The model under review builds one solid part; all positions refer to its coordinate system, in mm. A direction names the side the tool comes from. Coordinates: 2 decimals unless noted, no trailing zeros. Loops run counter-clockwise (first coordinate to the right, second up) from the corner with the lowest first, then second, coordinate; pieces in that order, holes last. Notation, with made-up numbers: M -19,12 L -5,12 A9 ccw -5,27 Z; hole C -11,-27.75 d5. An arc over 180 degrees is marked long. Use one line per item in the form item = value.
```python
from build123d import *

# Parameters (mm, degrees)
PAD_DEPTH       = 7
POCKET_DEPTH    = 0.5
POCKET001_DEPTH = 3
FILLET_R        = 2.99
PAD001_DEPTH    = 2
FILLET001_R     = 1.99
SKETCH004_R     = 0.275
PAD002_DEPTH    = 10


with BuildPart() as part:
    # Sketch → Pad (new body)
    with BuildSketch(Plane.XZ):
        with BuildLine():
            ThreePointArc((10, 5), (0, 15), (-10, 5))
            Line((-10, 5), (-10, -5))
            ThreePointArc((-10, -5), (0, -15), (10, -5))
            Line((10, 5), (10, -5))
        make_face()
    extrude(amount=PAD_DEPTH)

    # Sketch001 (on Face6 of Pad) → Pocket (cut)
    with BuildSketch(Plane.XZ.offset(7)):
        with BuildLine():
            ThreePointArc((9, 4.5), (0, 13.5), (-9, 4.5))
            Line((-9, 4.5), (-9, -4.5))
            ThreePointArc((-9, -4.5), (0, -13.5), (9, -4.5))
            Line((9, 4.5), (9, -4.5))
        make_face()
    extrude(amount=-POCKET_DEPTH, mode=Mode.SUBTRACT)

    # Sketch002 (on Face11 of Pocket) → Pocket001 (cut)
    with BuildSketch(Plane.XZ.offset(6.5)):
        with BuildLine():
            ThreePointArc((5, 4.5), (0, 9.5), (-5, 4.5))
            Line((-5, 4.5), (-5, -4.5))
            ThreePointArc((-5, -4.5), (0, -9.5), (5, -4.5))
            Line((5, 4.5), (5, -4.5))
        make_face()
    extrude(amount=-POCKET001_DEPTH, mode=Mode.SUBTRACT)

    # Fillet
    fillet_edges = [part.edges().sort_by_distance(p)[0] for p in [
        (0, -6.5, 9.5),
        (5, -6.5, 0),
        (-5, -6.5, 0),
        (0, -6.5, -9.5),
    ]]
    fillet(fillet_edges, radius=FILLET_R)

    # Sketch003 (on Face15 of Fillet) → Pad001 (join)
    with BuildSketch(Plane.XZ.offset(3.5)):
        with BuildLine():
            ThreePointArc((4, 4), (0, 8), (-4, 4))
            Line((-4, 4), (-4, -4))
            ThreePointArc((-4, -4), (0, -8), (4, -4))
            Line((4, 4), (4, -4))
        make_face()
    extrude(amount=PAD001_DEPTH)

    # Fillet001
    fillet001_edges = [part.edges().sort_by_distance(p)[0] for p in [
        (-4, -5.5, 0),
        (0, -5.5, -8),
        (4, -5.5, 0),
        (0, -5.5, 8),
    ]]
    fillet(fillet001_edges, radius=FILLET001_R)

    # Sketch004 (on DatumPlane) → Pad002 (join)
    with BuildSketch(Plane(origin=(0, -3.5, -11.366198), x_dir=(0, -1, 0), z_dir=(0, 0, 1))):
        with Locations((0.75, 0.375)):
            Circle(SKETCH004_R)
        with Locations((0.75, -0.375)):
            Circle(SKETCH004_R)
    extrude(amount=-PAD002_DEPTH)


solid = part.part
```
1. Add section D-D (z = -13). State the section outline as (x, y) points.
Response values:
outline = M -6,-7 L -2.96,-7 L -2.96,-6.5 L 2.96,-6.5 L 2.96,-7 L 6,-7 L 6,0 L -6,0 Z
2. Machinability: for faces 1 (the face through (9.6, -7, 0.1)), 2 (the face through (0, -5.5, 0)), which of the approach directions +Z, -Z, +X, -X, +Y, -Y give a long, thin tool a straight path to every point of the face, cutting with its end or side? Answer none if there is none.
Response values:
face_1 = +Z, -Z, +X, -X, -Y
face_2 = -Y
3. Add section C-C (y = -1.5). State the section outline as (x, z) points.
Response values:
outline = M -10,-5 A10 ccw 10,-5 L 10,5 A10 ccw -10,5 Z
4. Insertion check: P1, Ø3, axis at x = -2.5, z = -3, coming from the -Y side; P2, Ø1, axis at x = -2, y = -1.5, coming from the -Z side; P3, Ø1, axis at x = -5, z = 6.5, coming from the +Y side; P4, Ø9, axis at x = 1.5, z = 3.5, coming from the -Y side. Each pin has a flat end and moves straight along its axis. Give the tip position at first contact, or say it passes through.
Response values:
P1 = -5.5
P2 = -14.89
P3 = 0
P4 = -5.74
5. Wall thickness on line 1 along Y through (x, z) = (0, -3); line 2 along Z through (x, y) = (0.5, -3.75); line 3 along Z through (x, y) = (0.75, -3.75): over which ranges is each line inside the solid? List them lowest first. Write a range as from..to.
Response values:
line_1 = -5.5..0
line_2 = -14.99..-9.48, -7.95..7.95, 9.48..14.99
line_3 = -14.97..-9.45, -7.91..7.91, 9.45..14.97
6. Add section B-B (x = 8.5). State the section outline as (y, z) points.
Response values:
outline = M -7,-10.27 L 0,-10.27 L 0,10.27 L -7,10.27 L -7,7.46 L -6.5,7.46 L -6.5,-7.46 L -7,-7.46 Z
7. The part is to be moulded in two halves that separate along Z. For faces 3 (the face through (5.9, -5.65, 0.06)), 4 (the face through (0, -3, 15)), 5 (the face through (-10, -3, 0)), say which applies: pulls with the +Z half, pulls with the -Z half, needs draft (parallel to the pull), parting line crosses it, or undercut.
Response values:
face_3 = undercut
face_4 = pulls with the +Z half
face_5 = needs draft
